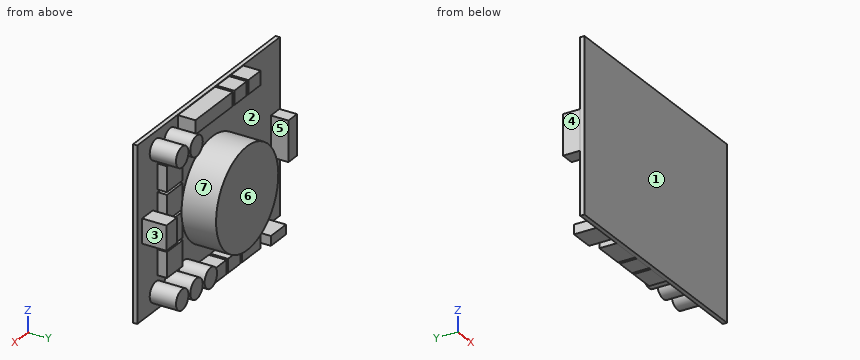
from build123d import *

# Parameters (mm, degrees)
SKETCH1_W           = 91.6
SKETCH1_H           = 68.7
BOSS_EXTRUDE1_DEPTH = 1.7
BOSS_EXTRUDE2_START = 4
SKETCH2_R           = 20
BOSS_EXTRUDE2_DEPTH = 13.8
SKETCH3_R           = 4
BOSS_EXTRUDE3_DEPTH = 10.5
SKETCH4_W           = 10
SKETCH4_H           = 10
BOSS_EXTRUDE4_DEPTH = 3.8
SKETCH6_R           = 10
BOSS_EXTRUDE5_DEPTH = 17.8
SKETCH7_W           = 6.8
SKETCH7_H           = 9.7
SKETCH7_W_2         = 9.7
SKETCH7_H_2         = 3.8
BOSS_EXTRUDE6_DEPTH = 9.7
SKETCH8_W           = 24
SKETCH8_H           = 5.5
SKETCH8_W_2         = 8
SKETCH8_W_3         = 5.5
SKETCH8_H_2         = 16
SKETCH8_W_4         = 12
SKETCH8_W_5         = 10
BOSS_EXTRUDE7_DEPTH = 7


with BuildPart() as part:
    # Sketch1 → Boss-Extrude1 (new body)
    with BuildSketch(Plane(origin=(0, 0, 0), x_dir=(1, 0, 0), z_dir=(0, 1, 0))):
        Rectangle(SKETCH1_W, SKETCH1_H)
    extrude(amount=BOSS_EXTRUDE1_DEPTH)

    # Sketch3 → Boss-Extrude3 (add)
    with BuildSketch(Plane(origin=(0, 1.7, 0), x_dir=(1, 0, 0), z_dir=(0, 1, 0))):
        with Locations(Location((15.4, 27.45, 0), (0, 0, 90))):
            Circle(SKETCH3_R)
        with Locations(Location((24.6, 27.45, 0), (0, 0, 90))):
            Circle(SKETCH3_R)
        with Locations(Location((33.8, 27.45, 0), (0, 0, 90))):
            Circle(SKETCH3_R)
        with Locations(Location((33.8, -27.45, 0), (0, 0, 90))):
            Circle(SKETCH3_R)
        with Locations(Location((24.6, -27.45, 0), (0, 0, 90))):
            Circle(SKETCH3_R)
    extrude(amount=BOSS_EXTRUDE3_DEPTH)

    # Sketch4 → Boss-Extrude4 (add)
    with BuildSketch(Plane(origin=(0, 1.7, 0), x_dir=(1, 0, 0), z_dir=(0, 1, 0))):
        with Locations((27.8, 5.5)):
            Rectangle(SKETCH4_W, SKETCH4_H)
        with Locations((27.8, 16.5)):
            Rectangle(SKETCH4_W, SKETCH4_H)
        with Locations((27.8, -5.5)):
            Rectangle(SKETCH4_W, SKETCH4_H)
        with Locations((27.8, -16.5)):
            Rectangle(SKETCH4_W, SKETCH4_H)
    extrude(amount=BOSS_EXTRUDE4_DEPTH)



with BuildPart() as body_2:
    # Sketch2 → Boss-Extrude2 (new body)
    with BuildSketch(Plane(origin=(0, 1.7, 0), x_dir=(1, 0, 0), z_dir=(0, 1, 0)).offset(BOSS_EXTRUDE2_START)):
        with Locations(Location((3.8, 0, 0), (0, 0, 270))):
            Circle(SKETCH2_R)
    extrude(amount=BOSS_EXTRUDE2_DEPTH)


with BuildPart() as part_1:
    add(part.part)

    add(body_2.part)  # Boss-Extrude5 merges body 2
    # Sketch6 → Boss-Extrude5 (add)
    with BuildSketch(Plane(origin=(0, 19.5, 0), x_dir=(1, 0, 0), z_dir=(0, 1, 0))):
        with Locations(Location((3.8, 0, 0), (0, 0, 270))):
            Circle(SKETCH6_R)
    extrude(amount=-BOSS_EXTRUDE5_DEPTH)

    # Sketch7 → Boss-Extrude6 (add)
    with BuildSketch(Plane(origin=(0, 1.7, 0), x_dir=(1, 0, 0), z_dir=(0, 1, 0))):
        with Locations((39.3, 0)):
            Rectangle(SKETCH7_W, SKETCH7_H)
        with Locations((-29.35, 31.6)):
            Rectangle(SKETCH7_W_2, SKETCH7_H_2)
    extrude(amount=BOSS_EXTRUDE6_DEPTH)

    # Sketch8 → Boss-Extrude7 (add)
    with BuildSketch(Plane(origin=(0, 1.7, 0), x_dir=(1, 0, 0), z_dir=(0, 1, 0))):
        with Locations((7.7, -31.4)):
            Rectangle(SKETCH8_W, SKETCH8_H)
        with Locations((-9.3, -31.4)):
            Rectangle(SKETCH8_W_2, SKETCH8_H)
        with Locations((-18.3, -31.4)):
            Rectangle(SKETCH8_W_2, SKETCH8_H)
        with Locations((-42.85, 1.15)):
            Rectangle(SKETCH8_W_3, SKETCH8_H_2)
        with Locations((-16.2, 31.4)):
            Rectangle(SKETCH8_W_4, SKETCH8_H)
        with Locations((-5.2, 31.4)):
            Rectangle(SKETCH8_W_2, SKETCH8_H)
        with Locations((4.8, 31.4)):
            Rectangle(SKETCH8_W_5, SKETCH8_H)
    extrude(amount=BOSS_EXTRUDE7_DEPTH)


solid = part_1.part
The model under review builds one solid part; all positions refer to its coordinate system, in mm. Face numbers are marked on the shaded views. A direction names the side the tool comes from. Coordinates: 2 decimals unless noted, no trailing zeros. Loops run counter-clockwise (first coordinate to the right, second up) from the corner with the lowest first, then second, coordinate; pieces in that order, holes last. Notation, with made-up numbers: M -4,23 L 28,23 A17 ccw 28,42 Z; hole C 84.25,17.25 d8. An arc over 180 degrees is marked long. Put each result on its own line as item: value. Start each with the question number.
Q1. The part is to be moulded in two halves that separate along Z. For the marked faces 1 and 2, say which applies: +Z half, -Z half, draft (parallel to the pull), parting line (faces both ways), or undercut.
Q2. Wall thickness on line 1 (Z direction, x = 3, y = 7.5); line 2 (X direction, y = 5.25, z = -8.5); line 3 (X direction, y = 2.25, z = 5.5): over which ranges is each line inside the solid? List them lowest first.
Q3. Clearance check with flat-ended pins moving along their axes: pin 1 (6.5 mm diameter, centred on x = 35, z = 27, fed in from +Y); pin 2 (3 mm diameter, centred on x = 14, y = 3.5, fed in from -Z); pin 3 (1.1 mm diameter, centred on x = -28.5, z = -31.5, fed in from +Y). State where each tip first meets the part, or that it passes through.
Q4. Add section C-C (x = 15.4). Write out the cut boundary in (y, z).
Q5. For the marked faces 3, 4, 5, 6 and 7, list the 3-axis set-ups (+Z, -Z, +X, -X, +Y, -Y) from which the entire face can be reached by the end or side of a thin tool; tool diameter is ignored.
Q6. Add section A-A (x = 3.8). Write out the cut boundary in (y, z).
Q7. Add section B-B (z = -19). Write out the cut boundary in (x, y) (3 decimals).
Q8. Add section D-D (z = -27.45). Write out the cut boundary in (x, y), and give its area (3 significant figures).
Answers:
1. face 1: draft
1. face 2: undercut
2. line 1: z = -34.15 to -28.65, -19.98 to 19.98, 28.65 to 34.15
2. line 2: x = -45.6 to -40.1, -1.47 to 9.07, 22.8 to 32.8
2. line 3: x = -45.6 to -40.1, -4.55 to 12.15, 22.8 to 32.8
3. pin 1: stops at y = 12.2
3. pin 2: stops at z = -31.45
3. pin 3: stops at y = 11.4
4. outline: M 0,-34.35 L 1.7,-34.35 L 1.7,-31.45 L 12.2,-31.45 L 12.2,-23.45 L 1.7,-23.45 L 1.7,28.65 L 8.7,28.65 L 8.7,34.15 L 1.7,34.15 L 1.7,34.35 L 0,34.35 Z; M 5.7,-16.29 L 19.5,-16.29 L 19.5,16.29 L 5.7,16.29 Z
5. face 3: +Z, -Z, +X, +Y
5. face 4: +Z, -Z, -X, +Y
5. face 5: +Z, -Z, +Y
5. face 6: +Z, -Z, +X, -X, +Y
5. face 7: +Y
6. outline: M 0,-34.35 L 1.7,-34.35 L 1.7,-34.15 L 8.7,-34.15 L 8.7,-28.65 L 1.7,-28.65 L 1.7,-10 L 5.7,-10 L 5.7,-20 L 19.5,-20 L 19.5,20 L 5.7,20 L 5.7,10 L 1.7,10 L 1.7,28.65 L 8.7,28.65 L 8.7,34.15 L 1.7,34.15 L 1.7,34.35 L 0,34.35 Z
7. outline: M -45.8,0 L 45.8,0 L 45.8,1.7 L 32.8,1.7 L 32.8,5.5 L 22.8,5.5 L 22.8,1.7 L -45.8,1.7 Z; M -2.445,5.7 L 10.045,5.7 L 10.045,19.5 L -2.445,19.5 Z
8. outline: M -45.8,0 L 45.8,0 L 45.8,1.7 L 37.8,1.7 L 37.8,12.2 L 29.8,12.2 L 29.8,1.7 L 28.6,1.7 L 28.6,12.2 L 20.6,12.2 L 20.6,1.7 L 19.4,1.7 L 19.4,12.2 L 11.4,12.2 L 11.4,1.7 L -45.8,1.7 Z
8. area: 408 mm^2
